The model under review builds one solid part; all positions refer to its coordinate system, in mm. A direction names the side the tool comes from. Round coordinates to 2 decimals unless told otherwise and drop trailing zeros. Order: outer loops, then holes, each group sorted by start corner. A loop starts at its lowest first (then second) coordinate and runs counter-clockwise, first axis right, second up.
```python
from build123d import *

# Parameters (mm, degrees)
SKETCH_5_R               = 4.25
EXTRUDE_5_DEPTH          = 30.5
CUT_EXTRUDE_2_DEPTH      = 63.121976788
CUT_EXTRUDE_5_DEPTH      = 42
CUT_EXTRUDE_5_DEPTH_BACK = 18
SKETCH_9_W               = 2
SKETCH_9_H               = 3


with BuildPart() as part:
    # 草图5 → 凸台-拉伸5 (new body)
    with BuildSketch(Plane(origin=(0, 0, 0), x_dir=(1, 0, 0), z_dir=(0, 1, 0))):
        with BuildLine():
            Line((-19.3, 0), (43.7, 0))
            ThreePointArc((43.7, 0), (49.356854249, -13.656854249), (35.7, -8))
            Line((35.7, -8), (35.7, -7))
            ThreePointArc((35.7, -7), (35.407106781, -6.292893219), (34.7, -6))
            Line((34.7, -6), (-10.3, -6))
            ThreePointArc((-10.3, -6), (-11.007106781, -6.292893219), (-11.3, -7))
            Line((-11.3, -7), (-11.3, -8))
            ThreePointArc((-11.3, -8), (-24.956854249, -13.656854249), (-19.3, 0))
        make_face()
        with Locations(Location((-19.3, -8, 0), (0, 0, 90))):
            Circle(SKETCH_5_R, mode=Mode.SUBTRACT)
        with Locations(Location((43.7, -8, 0), (0, 0, 90))):
            Circle(SKETCH_5_R, mode=Mode.SUBTRACT)
    extrude(amount=EXTRUDE_5_DEPTH)

    # 草图1 → 切除-拉伸2 (cut, through all)
    with BuildSketch(Plane.XY):
        with BuildLine():
            Line((24.2, 3), (26.9, 3))
            ThreePointArc((26.9, 3), (29.4, 5.5), (26.9, 8))
            Line((26.9, 8), (24.2, 8))
            ThreePointArc((24.2, 8), (21.7, 5.5), (24.2, 3))
        make_face()
        with BuildLine():
            Line((-2.5, 8), (0.2, 8))
            ThreePointArc((0.2, 8), (2.7, 5.5), (0.2, 3))
            Line((0.2, 3), (-2.5, 3))
            ThreePointArc((-2.5, 3), (-5, 5.5), (-2.5, 8))
        make_face()
        with BuildLine():
            Line((35.51684397, 5.5), (51.7, 5.5))
            Line((51.7, 5.5), (51.7, 0))
            Line((51.7, 0), (26.9, 0))
            ThreePointArc((26.9, 0), (29.859151728, 0.863900233), (31.88869914, 3.184210526))
            ThreePointArc((31.88869914, 3.184210526), (33.364733622, 4.871708922), (35.51684397, 5.5))
        make_face()
        with BuildLine():
            Line((-27.3, 5.5), (-11.11684397, 5.5))
            ThreePointArc((-11.11684397, 5.5), (-8.964733622, 4.871708922), (-7.48869914, 3.184210526))
            ThreePointArc((-7.48869914, 3.184210526), (-5.459151728, 0.863900233), (-2.5, 0))
            Line((-2.5, 0), (-27.3, 0))
            Line((-27.3, 0), (-27.3, 5.5))
        make_face()
        with BuildLine():
            Line((-11.3, 30.5), (-11.3, 17.5))
            ThreePointArc((-11.3, 17.5), (-9.835533906, 13.964466094), (-6.3, 12.5))
            Line((-6.3, 12.5), (30.7, 12.5))
            ThreePointArc((30.7, 12.5), (34.235533906, 13.964466094), (35.7, 17.5))
            Line((35.7, 17.5), (35.7, 30.5))
            Line((35.7, 30.5), (-11.3, 30.5))
        make_face()
    extrude(amount=CUT_EXTRUDE_2_DEPTH, mode=Mode.SUBTRACT)

    # 草图9 → 切除-拉伸5 (cut, two sides: drawn at the far end of the back side and taken through both)
    with BuildSketch(Plane(origin=(0, 0, 0), x_dir=(0, 0, -1), z_dir=(1, 0, 0)).offset(-CUT_EXTRUDE_5_DEPTH_BACK)):
        with Locations((-7, 6.523868095)):
            Rectangle(SKETCH_9_W, SKETCH_9_H)
    extrude(amount=CUT_EXTRUDE_5_DEPTH + CUT_EXTRUDE_5_DEPTH_BACK, mode=Mode.SUBTRACT)


solid = part.part
```
(1) To check wall thickness, follow probe 1 along X at (y, z) = (15, 8); probe 2 along Z at (x, y) = (-19, 16); probe 3 along X at (y, z) = (29, 6). State the ranges of each line that lie inside material, in increasing order.
Data:
probe 1: x = -27.3 to -23.55, -15.05 to -11.3, 35.7 to 39.45, 47.95 to 51.7
probe 2: z = 0 to 3.76, 12.24 to 15.99
probe 3: x = -27.05 to -23.05, -15.55 to -11.3, 35.7 to 39.95, 47.45 to 51.45
(2) Consider section A-A (y = 28). Write out the cut boundary in (x, z).
Data:
outline: (-19.3, 0) - (-11.3, 0) - (-11.3, 8) arc R8 ccw (long way) to start; (35.7, 0) - (43.7, 0) arc R8 ccw (long way) to (35.7, 8) - close; hole circle Ø8.5 at (-19.3, 8); hole circle Ø8.5 at (43.7, 8)
(3) Consider section C-C (x = 45). Write out the cut boundary in (y, z), and give its area (3 significant figures).
Data:
outline: (5.5, 0.11) - (30.5, 0.11) - (30.5, 3.95) - (5.5, 3.95) - close; (5.5, 12.05) - (30.5, 12.05) - (30.5, 15.89) - (5.5, 15.89) - close
area: 192 mm2
(4) Draft analysis for pull direction Z (two halves, no side actions). For faces 6 (the cylindrical face through (-24.77, 17.82, 13.84)), 7 (the flat face through (-14, 8.024, 7)), 8 (the cylindrical face through (-5.5, 0.89, 2.96)), state which applies: pulls with the +Z half, pulls with the -Z half, needs draft (parallel to the pull), parting line crosses it, or undercut.
Data:
face 6: parting line crosses it
face 7: undercut
face 8: needs draft
(5) Insertion check: pin 1 (6.5 mm diameter, centred on x = 13, z = 3.5, fed in from +Y); pin 2 (4.5 mm diameter, centred on x = 21, y = 6.5, fed in from +Z); pin 3 (8 mm diameter, centred on x = 47, z = 7, fed in from -Y); pin 4 (7 mm diameter, centred on x = 43.7, z = 8, fed in from -Y). Each pin has a flat end and moves straight along its axis. Give the tip position at first contact, or say it passes through.
Data:
pin 1: stops at y = 12.5
pin 2: stops at z = 6
pin 3: stops at y = 5.5
pin 4: passes through
(6) Consider section B-B (z = 14). Write out the cut boundary in (x, y).
Data:
outline: (-24.59, 5.5) - (-14.01, 5.5) - (-14.01, 30.5) - (-24.59, 30.5) - close; (38.41, 5.5) - (48.99, 5.5) - (48.99, 30.5) - (38.41, 30.5) - close
(7) Consider section D-D (y = 16.5). Write out the cut boundary in (x, z), and give its area (3 significant figures).
Data:
outline: (-19.3, 0) - (-11.2, 0) - (-11.2, 6.56) arc R1 cw to (-11.3, 7) - (-11.3, 8) arc R8 ccw (long way) to start; (35.6, 0) - (43.7, 0) arc R8 ccw (long way) to (35.7, 8) - (35.7, 7) arc R1 cw to (35.6, 6.56) - close; hole circle Ø8.5 at (-19.3, 8); hole circle Ø8.5 at (43.7, 8)
area: 317 mm2
(8) For faces 1 (the flat face through (-13, 7, 8)), 2 (the flat face through (-16, 5.5, 4)), 3 (the flat face through (47, 5.5, 4)), 4 (the cylindrical face through (21.7, 5.6, 3)), 5 (the flat face through (12, 12.5, 3)), list the 3-axis set-ups (+Z, -Z, +X, -X, +Y, -Y) from which the entire face can be reached by the end or side of a thin tool; tool diameter is ignored.
Data:
face 1: -Y
face 2: +Z, -Z, -X, -Y
face 3: +Z, -Z, +X, -Y
face 4: +Z, -Z
face 5: +Z, -Z, +Y
